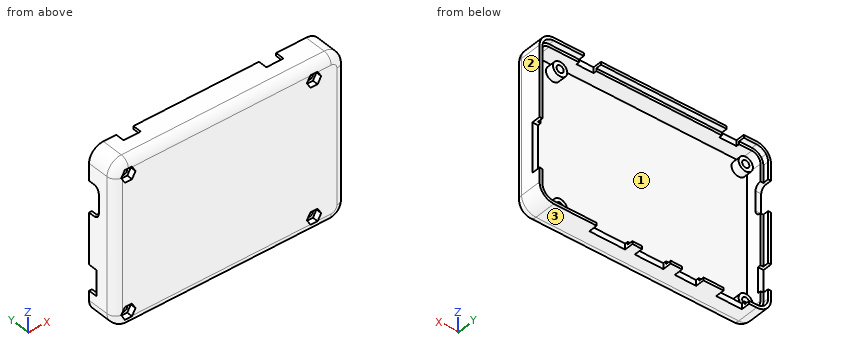
from build123d import *

# Parameters (mm, degrees)
SKETCH_4_W          = 81
SKETCH_4_H          = 57
SKETCH_4_R          = 1.25
EXTRUDE_5_DEPTH     = 3
EXTRUDE_START       = 3
SKETCH_4_4_R        = 2.5
SKETCH_4_4_R_2      = 1.25
EXTRUDE_6_DEPTH     = 3
SKETCH_4_5_W        = 81
SKETCH_4_5_H        = 57
SKETCH_4_5_W_2      = 77
SKETCH_4_5_H_2      = 53
EXTRUDE_7_DEPTH     = 10.6
SKETCH_6_W          = 12.5
SKETCH_6_H          = 3.1
SKETCH_6_W_2        = 10
SKETCH_6_W_3        = 7.5
SKETCH_6_W_4        = 9
CUT_EXTRUDE_1_DEPTH = 2
SKETCH_7_W          = 8.95
SKETCH_7_H          = 3.1
SKETCH_7_W_2        = 8.9
CUT_EXTRUDE_2_DEPTH = 2
FILLET_1_R          = 2
SKETCH_8_W          = 6
SKETCH_8_H          = 3.1
CUT_EXTRUDE_3_DEPTH = 2
SKETCH_9_W          = 17.3
SKETCH_9_H          = 3.1
CUT_EXTRUDE_4_DEPTH = 2
FILLET_2_R          = 3
FILLET_3_R          = 5
FILLET_4_R          = 3
CUT_EXTRUDE_5_DEPTH = 2
SKETCH_11_W         = 44
SKETCH_11_H         = 1
CUT_EXTRUDE_6_DEPTH = 2


with BuildPart() as part:
    # 草图4 → 凸台-拉伸5 (new body)
    with BuildSketch(Plane(origin=(0, 0, 0), x_dir=(1, 0, 0), z_dir=(0, 1, 0))):
        with Locations((-80.045972017, 113.056664423)):
            Rectangle(SKETCH_4_W, SKETCH_4_H)
        with Locations(Location((-115.545972017, 136.556664423, 0), (0, 0, 270))):
            Circle(SKETCH_4_R, mode=Mode.SUBTRACT)
        with Locations(Location((-50.545972017, 136.556664423, 0), (0, 0, 270))):
            Circle(SKETCH_4_R, mode=Mode.SUBTRACT)
        with Locations(Location((-50.545972017, 89.556664423, 0), (0, 0, 270))):
            Circle(SKETCH_4_R, mode=Mode.SUBTRACT)
        with Locations(Location((-115.545972017, 89.556664423, 0), (0, 0, 270))):
            Circle(SKETCH_4_R, mode=Mode.SUBTRACT)
    extrude(amount=EXTRUDE_5_DEPTH)

    # 草图4<4> → 凸台-拉伸6 (add)
    # profile 1 of 4: a face of its own
    with BuildSketch(Plane(origin=(0, 0, 0), x_dir=(1, 0, 0), z_dir=(0, 1, 0)).offset(EXTRUDE_START)):
        with Locations(Location((-50.545972017, 89.556664423, 0), (0, 0, 90))):
            Circle(SKETCH_4_4_R)
        with Locations(Location((-50.545972017, 89.556664423, 0), (0, 0, 90))):
            Circle(SKETCH_4_4_R_2, mode=Mode.SUBTRACT)
    # profile 2 of 4: a face of its own
    with BuildSketch(Plane(origin=(0, 0, 0), x_dir=(1, 0, 0), z_dir=(0, 1, 0)).offset(EXTRUDE_START)):
        with Locations(Location((-115.545972017, 89.556664423, 0), (0, 0, 90))):
            Circle(SKETCH_4_4_R)
        with Locations(Location((-115.545972017, 89.556664423, 0), (0, 0, 90))):
            Circle(SKETCH_4_4_R_2, mode=Mode.SUBTRACT)
    # profile 3 of 4: a face of its own
    with BuildSketch(Plane(origin=(0, 0, 0), x_dir=(1, 0, 0), z_dir=(0, 1, 0)).offset(EXTRUDE_START)):
        with Locations(Location((-50.545972017, 136.556664423, 0), (0, 0, 90))):
            Circle(SKETCH_4_4_R)
        with Locations(Location((-50.545972017, 136.556664423, 0), (0, 0, 90))):
            Circle(SKETCH_4_4_R_2, mode=Mode.SUBTRACT)
    # profile 4 of 4: a face of its own
    with BuildSketch(Plane(origin=(0, 0, 0), x_dir=(1, 0, 0), z_dir=(0, 1, 0)).offset(EXTRUDE_START)):
        with Locations(Location((-115.545972017, 136.556664423, 0), (0, 0, 90))):
            Circle(SKETCH_4_4_R)
        with Locations(Location((-115.545972017, 136.556664423, 0), (0, 0, 90))):
            Circle(SKETCH_4_4_R_2, mode=Mode.SUBTRACT)
    extrude(amount=EXTRUDE_6_DEPTH)

    # 草图4<5> → 凸台-拉伸7 (add)
    with BuildSketch(Plane(origin=(0, 0, 0), x_dir=(1, 0, 0), z_dir=(0, 1, 0))):
        with Locations((-80.045972017, 113.056664423)):
            Rectangle(SKETCH_4_5_W, SKETCH_4_5_H)
        with Locations((-80.045972017, 113.056664423)):
            Rectangle(SKETCH_4_5_W_2, SKETCH_4_5_H_2, mode=Mode.SUBTRACT)
    extrude(amount=EXTRUDE_7_DEPTH)

    # 草图6 → 切除-拉伸1 (cut)
    with BuildSketch(Plane(origin=(0, 0, -141.556664423), x_dir=(-1, 0, 0), z_dir=(0, 0, -1))):
        with Locations((65.795972017, 9.05)):
            Rectangle(SKETCH_6_W, SKETCH_6_H)
        with Locations((80.445972017, 9.05)):
            Rectangle(SKETCH_6_W_2, SKETCH_6_H)
        with Locations((93.195972017, 9.05)):
            Rectangle(SKETCH_6_W_3, SKETCH_6_H)
        with Locations((108.445972017, 9.05)):
            Rectangle(SKETCH_6_W_4, SKETCH_6_H)
    extrude(amount=-CUT_EXTRUDE_1_DEPTH, mode=Mode.SUBTRACT)

    # 草图7 → 切除-拉伸2 (cut)
    with BuildSketch(Plane.ZY.offset(120.545972017)):
        with Locations((-128.781664423, 9.05)):
            Rectangle(SKETCH_7_W, SKETCH_7_H)
        with Locations((-101.006664423, 9.05)):
            Rectangle(SKETCH_7_W_2, SKETCH_7_H)
        Polygon((-105.456664423, 10.6), (-106.456664423, 10.6), (-106.456664423, 6.5), (-95.556664423, 6.5), (-95.556664423, 10.6), (-96.556664423, 10.6), (-96.556664423, 7.5), (-105.456664423, 7.5), align=None)
    extrude(amount=-CUT_EXTRUDE_2_DEPTH, mode=Mode.SUBTRACT)

    # 圆角1
    fillet_1_edges = [part.edges().sort_by_distance(p)[0] for p in [
        (-119.545972017, 6.5, -95.556664423),
        (-119.545972017, 6.5, -106.456664423),
    ]]
    fillet(fillet_1_edges, radius=FILLET_1_R)

    # 草图8 → 切除-拉伸3 (cut)
    with BuildSketch(Plane.XY.offset(-84.556664423)):
        with Locations((-108.045972017, 9.05)):
            Rectangle(SKETCH_8_W, SKETCH_8_H)
        with Locations((-58.045972017, 9.05)):
            Rectangle(SKETCH_8_W, SKETCH_8_H)
    extrude(amount=-CUT_EXTRUDE_3_DEPTH, mode=Mode.SUBTRACT)

    # 草图9 → 切除-拉伸4 (cut)
    with BuildSketch(Plane(origin=(-39.545972017, 0, 0), x_dir=(0, 0, -1), z_dir=(1, 0, 0))):
        with Locations((122.906664423, 9.05)):
            Rectangle(SKETCH_9_W, SKETCH_9_H)
    extrude(amount=-CUT_EXTRUDE_4_DEPTH, mode=Mode.SUBTRACT)

    # 圆角2
    fillet_2_edges = [part.edges().sort_by_distance(p)[0] for p in [
        (-118.545972017, 6.8, -139.556664423),
        (-41.545972017, 6.8, -139.556664423),
        (-41.545972017, 6.8, -86.556664423),
        (-118.545972017, 6.8, -86.556664423),
    ]]
    fillet(fillet_2_edges, radius=FILLET_2_R)

    # 圆角3
    fillet_3_edges = [part.edges().sort_by_distance(p)[0] for p in [
        (-120.545972017, 5.3, -141.556664423),
        (-120.545972017, 5.3, -84.556664423),
        (-39.545972017, 5.3, -84.556664423),
        (-39.545972017, 5.3, -141.556664423),
    ]]
    fillet(fillet_3_edges, radius=FILLET_3_R)

    # 圆角4
    fillet_4_edges = [part.edges().sort_by_distance(p)[0] for p in [
        (-80.045972017, 0, -84.556664423),
        (-80.045972017, 0, -141.556664423),
        (-39.545972017, 0, -113.056664423),
        (-120.545972017, 0, -113.056664423),
        (-119.081505923, 0, -140.092198329),
        (-41.010438111, 0, -140.092198329),
        (-41.010438111, 0, -86.021130517),
        (-119.081505923, 0, -86.021130517),
    ]]
    fillet(fillet_4_edges, radius=FILLET_4_R)

    # 草图10 → 切除-拉伸5 (cut)
    with BuildSketch(Plane.XZ):
        Polygon((-48.045972017, -89.556664423), (-49.295972017, -87.391600913), (-51.795972017, -87.391600913), (-53.045972017, -89.556664423), (-51.795972017, -91.721727932), (-49.295972017, -91.721727932), align=None)
        Polygon((-113.045972017, -89.556664423), (-114.295972017, -87.391600913), (-116.795972017, -87.391600913), (-118.045972017, -89.556664423), (-116.795972017, -91.721727932), (-114.295972017, -91.721727932), align=None)
        Polygon((-113.045972017, -136.556664423), (-114.295972017, -134.391600913), (-116.795972017, -134.391600913), (-118.045972017, -136.556664423), (-116.795972017, -138.721727932), (-114.295972017, -138.721727932), align=None)
        Polygon((-48.045972017, -136.556664423), (-49.295972017, -134.391600913), (-51.795972017, -134.391600913), (-53.045972017, -136.556664423), (-51.795972017, -138.721727932), (-49.295972017, -138.721727932), align=None)
    extrude(amount=-CUT_EXTRUDE_5_DEPTH, mode=Mode.SUBTRACT)

    # 草图11 → 切除-拉伸6 (cut)
    with BuildSketch(Plane(origin=(0, 10.6, 0), x_dir=(1, 0, 0), z_dir=(0, 1, 0))):
        with BuildLine():
            Line((-41.261655488, 87.273406895), (-42.082349142, 87.844775895))
            ThreePointArc((-42.082349142, 87.844775895), (-43.155947841, 86.898124825), (-44.545972017, 86.556664423))
            Line((-44.545972017, 86.556664423), (-61.045972017, 86.556664423))
            Line((-61.045972017, 86.556664423), (-61.045972017, 85.556664423))
            Line((-61.045972017, 85.556664423), (-44.545972017, 85.556664423))
            ThreePointArc((-44.545972017, 85.556664423), (-42.693005491, 86.011736348), (-41.261655488, 87.273406895))
        make_face()
        with BuildLine():
            ThreePointArc((-40.545972017, 136.556664423), (-41.168680103, 138.700002783), (-42.842921681, 140.17600408))
            Line((-42.842921681, 140.17600408), (-43.850059004, 139.474832526))
            ThreePointArc((-43.850059004, 139.474832526), (-42.1914297, 138.415731522), (-41.545972017, 136.556664423))
            Line((-41.545972017, 136.556664423), (-41.545972017, 89.556664423))
            ThreePointArc((-41.545972017, 89.556664423), (-41.683205119, 88.659688566), (-42.082349142, 87.844775895))
            Line((-42.082349142, 87.844775895), (-41.261655488, 87.273406895))
            ThreePointArc((-41.261655488, 87.273406895), (-40.729084141, 88.360266938), (-40.545972017, 89.556664423))
            Line((-40.545972017, 89.556664423), (-40.545972017, 136.556664423))
        make_face()
        with BuildLine():
            Line((-44.545972017, 140.556664423), (-115.545972017, 140.556664423))
            ThreePointArc((-115.545972017, 140.556664423), (-116.418508942, 140.460339526), (-117.249022353, 140.17600408))
            Line((-117.249022353, 140.17600408), (-116.24188503, 139.474832526))
            ThreePointArc((-116.24188503, 139.474832526), (-115.896325903, 139.536136214), (-115.545972017, 139.556664423))
            Line((-115.545972017, 139.556664423), (-44.545972017, 139.556664423))
            ThreePointArc((-44.545972017, 139.556664423), (-44.195618131, 139.536136214), (-43.850059004, 139.474832526))
            Line((-43.850059004, 139.474832526), (-42.842921681, 140.17600408))
            ThreePointArc((-42.842921681, 140.17600408), (-43.673435092, 140.460339526), (-44.545972017, 140.556664423))
        make_face()
        with BuildLine():
            Line((-116.24188503, 139.474832526), (-117.249022353, 140.17600408))
            ThreePointArc((-117.249022353, 140.17600408), (-118.923263931, 138.700002783), (-119.545972017, 136.556664423))
            Line((-119.545972017, 136.556664423), (-119.545972017, 89.556664423))
            ThreePointArc((-119.545972017, 89.556664423), (-119.362859893, 88.360266938), (-118.830288546, 87.273406895))
            Line((-118.830288546, 87.273406895), (-118.009594892, 87.844775895))
            ThreePointArc((-118.009594892, 87.844775895), (-118.408738915, 88.659688566), (-118.545972017, 89.556664423))
            Line((-118.545972017, 89.556664423), (-118.545972017, 136.556664423))
            ThreePointArc((-118.545972017, 136.556664423), (-117.900514333, 138.415731522), (-116.24188503, 139.474832526))
        make_face()
        with BuildLine():
            ThreePointArc((-115.545972017, 86.556664423), (-116.935996192, 86.898124825), (-118.009594892, 87.844775895))
            Line((-118.009594892, 87.844775895), (-118.830288546, 87.273406895))
            ThreePointArc((-118.830288546, 87.273406895), (-117.398938542, 86.011736348), (-115.545972017, 85.556664423))
            Line((-115.545972017, 85.556664423), (-105.045972017, 85.556664423))
            Line((-105.045972017, 85.556664423), (-105.045972017, 86.556664423))
            Line((-105.045972017, 86.556664423), (-115.545972017, 86.556664423))
        make_face()
        with Locations((-83.045972017, 86.056664423)):
            Rectangle(SKETCH_11_W, SKETCH_11_H)
    extrude(amount=-CUT_EXTRUDE_6_DEPTH, mode=Mode.SUBTRACT)


solid = part.part
Read the model definition and answer for the solid it produces. Units are mm, in the model's axes. Face numbers are marked on the shaded views. Coordinates: 2 decimals unless noted, no trailing zeros. Write each loop counter-clockwise with the first axis right and the second up, starting at its lowest first coordinate (ties: lowest second). Pieces come first, ordered by that corner, then holes. Notation, with made-up numbers: M 31.5,51 L 83.5,51 A26 ccw 83.5,84 Z; hole C -9,-39 d3. An arc over 180 degrees is marked long. Use a Markdown table: item, result.
Q1. The part is cut by section A-A, the plane z = -130. Write down the section's boundary in (x, y).
Answer block:
| item | result |
|---|---|
| outline | M -120.55,3 A3 ccw -117.55,0 L -42.55,0 A3 ccw -39.55,3 L -39.55,7.5 L -41.55,7.5 L -41.55,3 L -118.55,3 L -118.55,7.5 L -120.55,7.5 Z |
Q2. The part is cut by section C-C, the plane y = 9.75. Give the number of separate pieces and of enclosed holes in the cut face, then the cut area to 3 significant figures.
Answer block:
| item | result |
|---|---|
| separate pieces | 9 |
| enclosed holes | 0 |
| area | 176 mm2 |
Q3. The part is cut by section B-B, the plane x = -109. Write down the section's boundary in (y, z), then the cut area to 3 significant figures.
Answer block:
| item | result |
|---|---|
| outline | M 0,-138.56 A3 ccw 3,-141.56 L 7.5,-141.56 L 7.5,-139.56 L 3,-139.56 L 3,-86.56 L 7.5,-86.56 L 7.5,-84.56 L 3,-84.56 A3 ccw 0,-87.56 Z |
| area | 185 mm2 |
Q4. Straight lines are drawn through the part: L1, parallel to X at y = 6.75, z = -127.5; L2, parallel to Z at x = -114.5, y = 9.5; L3, parallel to Z at x = -64.5, y = 6.5. For each, find the intervals that lie inside material, in ascending order. Write a range as [from, to].
Answer block:
| item | result |
|---|---|
| L1 | x = [-120.55, -118.55], [-41.55, -39.55] |
| L2 | z = [-141.56, -140.56], [-85.56, -84.56] |
| L3 | z = [-141.56, -139.56], [-86.56, -84.56] |
Q5. Each of these flat-tipped pins is pushed along its axis until it touches: pin 1 Ø2 at (y, z) = (9, -141) entering from +X; pin 2 Ø1 at (x, z) = (-119.5, -99.5) entering from +Y; pin 3 Ø1.6 at (x, y) = (-116, 1.5) entering from +Z. Where does it stop, or does it pass through?
Answer block:
| item | result |
|---|---|
| pin 1 | stops at x = -40.92 |
| pin 2 | stops at y = 6.5 |
| pin 3 | stops at z = -84.65 |
Q6. The part is cut by section D-D, the plane z = -123. Write down the section's boundary in (x, y), then the cut area to 3 significant figures.
Answer block:
| item | result |
|---|---|
| outline | M -120.55,3 A3 ccw -117.55,0 L -42.55,0 A3 ccw -39.55,3 L -39.55,7.5 L -41.55,7.5 L -41.55,3 L -118.55,3 L -118.55,8.6 L -119.55,8.6 L -119.55,10.6 L -120.55,10.6 Z |
| area | 261 mm2 |
Q7. Determine the mould class of the marked faces 1, 2 and 3 for opening direction X: released by +X, released by -X, zero draft, split by the parting line, or undercut.
Answer block:
| item | result |
|---|---|
| face 1 | undercut |
| face 2 | released by +X |
| face 3 | zero draft |
